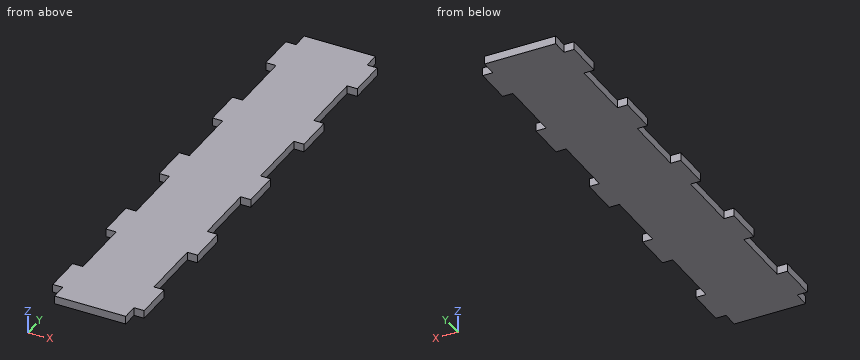
from build123d import *

# Parameters (mm, degrees)
SKETCH1_W          = 36
SKETCH1_H          = 200
BASE_FLANGE1_DEPTH = 3.175
SKETCH2_W          = 4
SKETCH2_H          = 25
CUT_EXTRUDE1_DEPTH = 10
LPATTERN1_COUNT    = 6
LPATTERN1_PITCH    = 40
SKETCH3_W          = 28
SKETCH3_H          = 6.25
CUT_EXTRUDE2_DEPTH = 10


# Sheet-metal steps are written as plain solids
with BuildPart() as part:
    # Sketch1 → Base-Flange1 (new body)
    with BuildSketch(Plane.XY):
        with Locations((25.081146731, 10.708830738)):
            Rectangle(SKETCH1_W, SKETCH1_H)
    extrude(amount=-BASE_FLANGE1_DEPTH)

    # Sketch2 → Cut-Extrude1 (cut)
    with BuildSketch(Plane.XY):
        with Locations((9.081146731, -89.291169262)):
            Rectangle(SKETCH2_W, SKETCH2_H)
        with Locations((41.081146731, -89.291169262)):
            Rectangle(SKETCH2_W, SKETCH2_H)
    cut_extrude1 = extrude(amount=-CUT_EXTRUDE1_DEPTH, mode=Mode.SUBTRACT)

    # LPattern1: Cut-Extrude1 ×6
    with Locations(*[(0, i * LPATTERN1_PITCH, 0) for i in range(1, LPATTERN1_COUNT)]):
        add(cut_extrude1, mode=Mode.SUBTRACT)

    # Sketch3 → Cut-Extrude2 (cut)
    with BuildSketch(Plane.XY):
        with Locations((25.081146731, 107.583830738)):
            Rectangle(SKETCH3_W, SKETCH3_H)
        with Locations((25.081146731, -86.166169262)):
            Rectangle(SKETCH3_W, SKETCH3_H)
    extrude(amount=-CUT_EXTRUDE2_DEPTH, mode=Mode.SUBTRACT)


solid = part.part
For this review, take the finished solid that the model builds, in its own axes (mm). Round coordinates to 2 decimals unless told otherwise and drop trailing zeros. Loops run counter-clockwise (first coordinate to the right, second up) from the corner with the lowest first, then second, coordinate; pieces in that order, holes last. Notation, with made-up numbers: (-17, -40) - (8, -40) arc R19 ccw to (8, -9) - close; hole circle Ø9 at (-11.5, 26). An arc over 180 degrees is marked (long way). Answer as CSV lines item,"result".
(1) Wall thickness on line 1 (Y direction, x = 39.5, z = -1.9); line 2 (X direction, y = -60, z = -0.85): over which ranges is each line inside the solid? List them lowest first.
Checked values:
line 1,"y = -76.79 to -61.79, -36.79 to -21.79, 3.21 to 18.21, 43.21 to 58.21, 83.21 to 98.21"
line 2,"x = 11.08 to 39.08"
(2) Consider section A-A on y = 78. Give the boundary of the cut face in (x, z) (3 decimals).
Checked values:
outline,"(11.081, -3.175) - (39.081, -3.175) - (39.081, 0) - (11.081, 0) - close"
(3) Insertion check: P1, Ø1.6, axis at x = 8.5, z = -1, coming from the -Y side; P2, Ø1, axis at y = 30.5, z = -1.5, coming from the -X side; P3, Ø1.6, axis at x = 42, z = -1.5, coming from the +Y side. Each pin has a flat end and moves straight along its axis. Give the tip position at first contact, or say it passes through.
Checked values:
P1,"stops at y = -76.79"
P2,"stops at x = 11.08"
P3,"stops at y = 98.21"
